Geometry: final body of the model. Coordinates: model frame, mm. Face numbers are marked on the shaded views. A direction names the side the tool comes from. Give positions to 0.01 mm unless a question says otherwise; leave off trailing zeros. Write each loop counter-clockwise with the first axis right and the second up, starting at its lowest first coordinate (ties: lowest second). Pieces come first, ordered by that corner, then holes.
```python
from build123d import *

# Parameters (mm, degrees)
F0_W      = 70
F0_H      = 2.5
F1_DEPTH  = 150
F2_W      = 52.524413
F2_H      = 110
F3_DEPTH  = 2.501
F4_W      = 110
F4_H      = 30
F5_DEPTH  = 17.506528
F6_DEPTH  = 74.667651
F7_R      = 2
F8_DEPTH  = 1.5
F9_R      = 3.75
F10_R     = 3.75
F11_DEPTH = 2
F12_R     = 15
F13_R     = 15
F14_R     = 5


with BuildPart() as f1:
    # F0 (on Front) → F1 (new body)
    with BuildSketch(Plane.XZ):
        Rectangle(F0_W, F0_H)
        with BuildLine():
            Line((-35, -1.25), (-35, 1.25))
            ThreePointArc((-35, 1.25), (-36.438277, 1.617252), (-37.524413, 2.629093))
            Line((-37.524413, 2.629093), (-39.62809, 1.278337))
            ThreePointArc((-39.62809, 1.278337), (-37.63684, -0.576704), (-35, -1.25))
        make_face()
        Polygon((-39.62809, 1.278337), (-37.524413, 2.629093), (-53.733482, 27.873223), (-55.83716, 26.522467), align=None)
    extrude(amount=F1_DEPTH)

    # F2 (on face) → F3 (cut, through all)
    with BuildSketch(Plane.XY.offset(1.25)):
        with Locations((-11.262206, -75)):
            Rectangle(F2_W, F2_H)
    extrude(amount=-F3_DEPTH, mode=Mode.SUBTRACT)

    # F4 (on face) → F5 (cut, through all)
    with BuildSketch(Plane(origin=(-25.374726, 0, -16.292924), x_dir=(0, 1, 0), z_dir=(0.841471, 0, 0.540302))):
        with Locations((-75, 17.486832)):
            Rectangle(F4_W, F4_H)
    extrude(amount=-F5_DEPTH, mode=Mode.SUBTRACT)

    # F4 (on face) → F6 (cut, through all)
    with BuildSketch(Plane(origin=(-25.374726, 0, -16.292924), x_dir=(0, 1, 0), z_dir=(0.841471, 0, 0.540302))):
        with Locations((-75, 17.486832)):
            Rectangle(F4_W, F4_H)
    extrude(amount=F6_DEPTH, mode=Mode.SUBTRACT)

    # F7 (on face) → F8 (join)
    with BuildSketch(Plane(origin=(-27.478403, 0, -17.64368), x_dir=(0, -1, 0), z_dir=(-0.841471, 0, -0.540302))):
        with Locations((10.75, 32.486832)):
            Circle(F7_R)
        with Locations((139.25, 32.486832)):
            Circle(F7_R)
    extrude(amount=F8_DEPTH)

    # F9 (on face) + F10 (on face) → F11 (join)
    with BuildSketch(Plane(origin=(-28.74061, 0, -18.454133), x_dir=(0, -1, 0), z_dir=(-0.841471, 0, -0.540302))):
        with Locations((10.75, 32.486832)):
            Circle(F9_R)
    with BuildSketch(Plane(origin=(-28.74061, 0, -18.454133), x_dir=(0, -1, 0), z_dir=(-0.841471, 0, -0.540302))):
        with Locations((139.25, 32.486832)):
            Circle(F10_R)
    extrude(amount=F11_DEPTH)

    # F12
    f12_edges = [f1.edges().sort_by_distance(p)[0] for p in [
        (-54.785321, 0, 27.197845),
    ]]
    fillet(f12_edges, radius=F12_R)

    # F13
    f13_edges = [f1.edges().sort_by_distance(p)[0] for p in [
        (-54.785321, -150, 27.197845),
        (35, -150, 0),
        (35, 0, 0),
    ]]
    fillet(f13_edges, radius=F13_R)

    # F14
    f14_edges = [f1.edges().sort_by_distance(p)[0] for p in [
        (-43.979275, -20, 10.368425),
        (15, -20, 0),
        (15, -130, 0),
        (-43.979275, -130, 10.368425),
    ]]
    fillet(f14_edges, radius=F14_R)


solid = f1.part
```
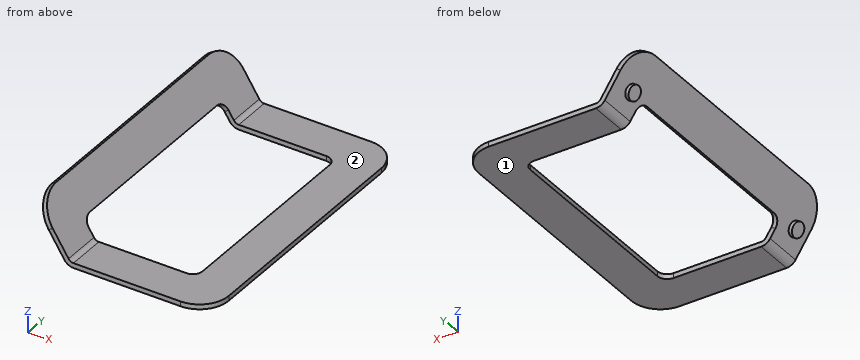
Item 1: Section B-B, the plane x = -22.5. Return the cut outline in (y, z), plus the area to 3 significant figures.
Found:
outline: (-150, -1.25) - (-130, -1.25) - (-130, 1.25) - (-150, 1.25) - close; (-20, -1.25) - (0, -1.25) - (0, 1.25) - (-20, 1.25) - close
area: 100 mm2
Item 2: Section A-A, the plane y = -38.5. Return the cut outline in (x, z), plus the area to 3 significant figures.
Found:
outline: (-55.84, 26.52) - (-45.03, 9.69) - (-42.93, 11.04) - (-53.73, 27.87) - close; (15, -1.25) - (35, -1.25) - (35, 1.25) - (15, 1.25) - close
area: 100 mm2
Item 3: Line query: L1, parallel to Y at x = -34, z = 0.5; L2, parallel to Z at x = 22, y = -54. Output: solid intervals per line, ascending.
Found:
L1: y = -150 to -130, -20 to 0
L2: z = -1.25 to 1.25
Item 4: Section D-D, the plane x = 16.5. Return the cut outline in (y, z).
Found:
outline: (-150, -1.25) - (0, -1.25) - (0, 1.25) - (-150, 1.25) - close
Item 5: Reachability of the marked faces 1 and 2 from +Z, -Z, +X, -X, +Y, -Y: full face, straight path, thin tool, end or side. Return the list, or none.
Found:
face 1: -Z, +X, -X, +Y, -Y
face 2: +Z, +X, +Y, -Y
Item 6: Pin query (flat end, axial travel): pin 1 Ø0.8 at (y, z) = (-72.5, -0.5) entering from -X; pin 2 Ø1 at (x, z) = (-21.5, 2.5) entering from -Y (3 decimals); pin 3 Ø21 at (x, y) = (11, -45.5) entering from +Z. Return the tip coordinate at first contact, or that it passes through.
Found:
pin 1: stops at x = 15
pin 2: passes through
pin 3: stops at z = 1.25
Item 7: Section C-C, the plane y = -17. Return the cut outline in (x, z), plus the area to 3 significant figures.
Found:
outline: (-55.84, 26.52) - (-39.63, 1.28) arc R5.5 ccw to (-35, -1.25) - (35, -1.25) - (35, 1.25) - (-35, 1.25) arc R3 cw to (-37.52, 2.63) - (-53.73, 27.87) - close
area: 261 mm2
